Source: three-view drawing plus pictorial views. Frame: mm from the lowest corner of the part. Round coordinates to 2 decimals unless told otherwise and drop trailing zeros. Loops run counter-clockwise (first coordinate to the right, second up) from the corner with the lowest first, then second, coordinate; pieces in that order, holes last. Notation, with made-up numbers: M 5.25,9.25 L 22.25,9.25 A23 cw 22.25,30.25 Z; hole C 60.25,49 d10. An arc over 180 degrees is marked long. Write each question's results on one line, items separated by ' | '.
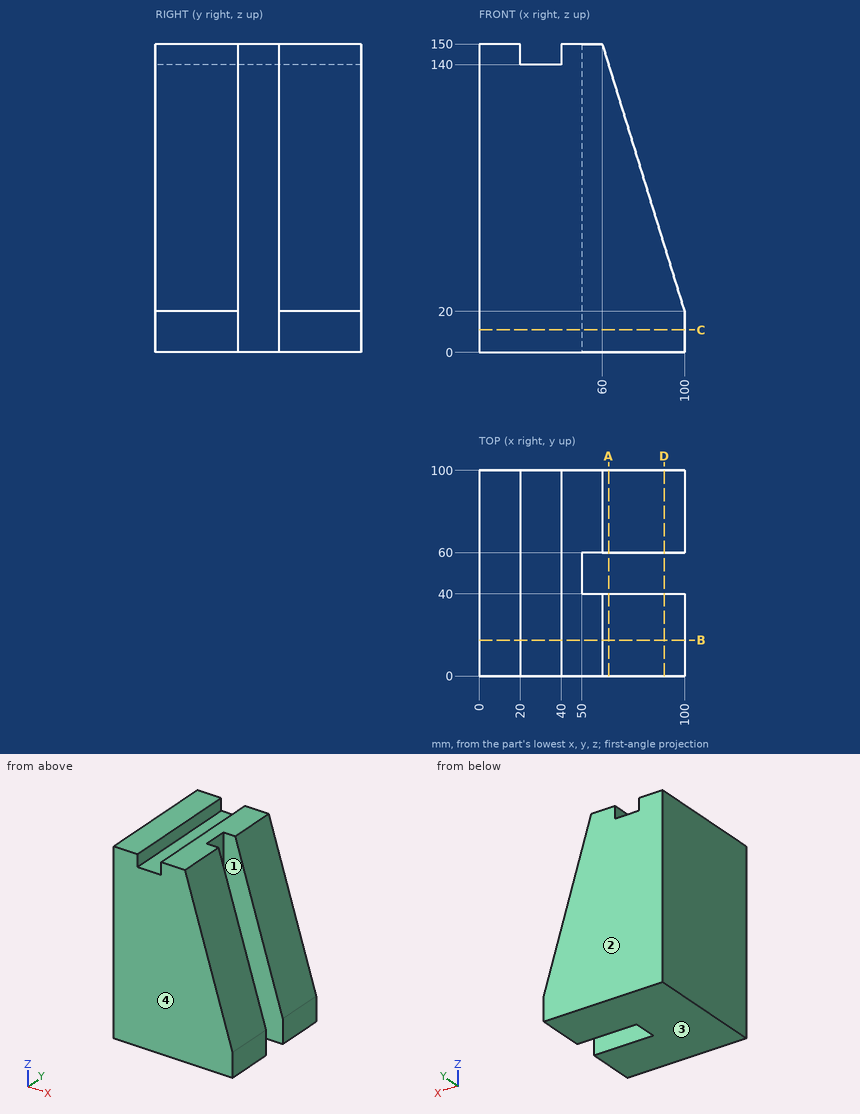
1. Section D-D (x = 90). Output: boundary loops of the cut face in (y, z), then the cut area to 3 significant figures.
Answer key:
outline: M 0,0 L 40,0 L 40,52.5 L 0,52.5 Z; M 60,0 L 100,0 L 100,52.5 L 60,52.5 Z | area: 4,200 mm²
2. Section A-A (x = 63). Output: boundary loops of the cut face in (y, z), then the cut area to 3 significant figures.
Answer key:
outline: M 0,0 L 40,0 L 40,140.25 L 0,140.25 Z; M 60,0 L 100,0 L 100,140.25 L 60,140.25 Z | area: 11,200 mm²
3. Section B-B (y = 17.5). Output: boundary loops of the cut face in (x, z).
Answer key:
outline: M 0,0 L 100,0 L 100,20 L 60,150 L 40,150 L 40,140 L 20,140 L 20,150 L 0,150 Z
4. Pin query (flat end, axial travel): P1, Ø5, axis at y = 43, z = 144, coming from the +X side; P2, Ø22, axis at y = 48, z = 66, coming from the +X side. Return the tip coordinate at first contact, or that it passes through.
Answer key:
P1: stops at x = 50 | P2: stops at x = 88.17
5. Ray query, probe 1 along Y at (x, z) = (85, 42); probe 2 along Z at (x, y) = (36, 80); probe 3 along X at (y, z) = (48, 64). Return the intervals inside material, ascending.
Answer key:
probe 1: y = 0 to 40, 60 to 100 | probe 2: z = 0 to 140 | probe 3: x = 0 to 50
6. Section C-C (z = 11). Output: boundary loops of the cut face in (x, y), then the cut area to 3 significant figures.
Answer key:
outline: M 0,0 L 100,0 L 100,40 L 50,40 L 50,60 L 100,60 L 100,100 L 0,100 Z | area: 9,000 mm²
7. Draft query along Y for the marked faces 1, 2, 3 and 4. Return one class per face: pulls with the +Y half, pulls with the -Y half, needs draft (parallel to the pull), parting line crosses it, or undercut.
Answer key:
face 1: undercut | face 2: pulls with the +Y half | face 3: needs draft | face 4: pulls with the -Y half
